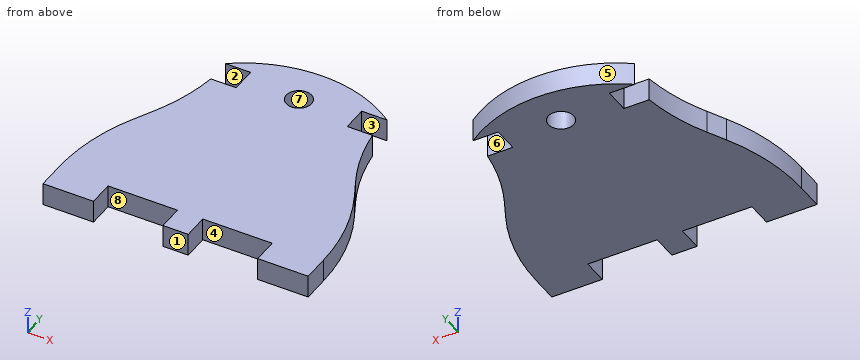
```python
from build123d import *

# Parameters (mm, degrees)
SKETCH1_R           = 2.5
BOSS_EXTRUDE1_DEPTH = 4.5
FILLET1_R           = 40
SKETCH2_W           = 5
SKETCH2_H           = 4.5
BOSS_EXTRUDE2_DEPTH = 5
CHAMFER1_SIZE       = 6
FILLET2_R           = 30
CUT_EXTRUDE1_DEPTH  = 10


# Some blends are built 0.0001 mm under size
with BuildPart() as part:
    # Sketch1 → Boss-Extrude1 (new body)
    with BuildSketch(Plane.XY):
        Polygon((-16.25, 10.704231142), (-16.25, 15.704231142), (16.25, 15.704231142), (16.25, 10.704231142), (26.25, 10.704231142), (26.25, 25.704231142), (16, 45.704231142), (16, 50.704231142), (11, 50.704231142), (11, 55.704231142), (16, 55.704231142), (16, 61.704231142), (-16, 61.704231142), (-16, 55.704231142), (-11, 55.704231142), (-11, 50.704231142), (-16, 50.704231142), (-16, 45.704231142), (-26.25, 25.704231142), (-26.25, 10.704231142), align=None)
        with Locations((0, 53.212370659)):
            Circle(SKETCH1_R, mode=Mode.SUBTRACT)
    extrude(amount=BOSS_EXTRUDE1_DEPTH)

    # Fillet1
    # the kernel refuses this fillet: 40 mm, written as the material it adds along each edge
    with BuildSketch(Plane(origin=(-16, 45.704231142, 0), x_dir=(0, 1, 0), z_dir=(0, 0, 1))) as fillet1_piece_1:
        with BuildLine():
            CenterArc((10.355860331, 39.639812816), FILLET1_R, 242.864860378, 19.440324463)
            Line((-7.887771306, 4.042482794), (0, 0))
            Line((0, 0), (5, 0))
        make_face()
    extrude(amount=4.5)
    with BuildSketch(Plane(origin=(16, 45.704231142, 0), x_dir=(0.4560907909103989, -0.8899332505568757, 0), z_dir=(0, 0, 1))) as fillet1_piece_2:
        with BuildLine():
            CenterArc((8.863329132, 40), FILLET1_R, 250.559675537, 19.440324463)
            Line((-4.449666253, 2.280453955), (0, 0))
            Line((0, 0), (8.863329132, 0))
        make_face()
    extrude(amount=4.5)
    # the kernel refuses this fillet: 40 mm, written as the material it takes off along each edge
    with BuildSketch(Plane(origin=(-26.25, 25.704231142, -24.132640175), x_dir=(0, -1, 0), z_dir=(0, 0, 1))) as fillet1_2_piece_1:
        with BuildLine():
            CenterArc((FILLET1_R * 0.241326401753, FILLET1_R), FILLET1_R, 242.864860378, 27.135139622)
            Line((-FILLET1_R * 0.214764389157, FILLET1_R * 0.110066749443), (0, 0))
            Line((0, 0), (FILLET1_R * 0.241326401753, 0))
        make_face()
    extrude(amount=52.765280351, mode=Mode.SUBTRACT)
    with BuildSketch(Plane(origin=(26.25, 25.704231142, -24.132640175), x_dir=(0, -1, 0), z_dir=(0, 0, 1))) as fillet1_2_piece_2:
        with BuildLine():
            CenterArc((FILLET1_R * 0.241326401753, -FILLET1_R), FILLET1_R, 90, 27.135139622)
            Line((-FILLET1_R * 0.214764389157, -FILLET1_R * 0.110066749443), (0, 0))
            Line((0, 0), (FILLET1_R * 0.241326401753, 0))
        make_face()
    extrude(amount=52.765280351, mode=Mode.SUBTRACT)

    # Sketch2 → Boss-Extrude2 (add)
    with BuildSketch(Plane.XZ.offset(-15.704231142)):
        with Locations((0, 2.25)):
            Rectangle(SKETCH2_W, SKETCH2_H)
    extrude(amount=BOSS_EXTRUDE2_DEPTH)

    # Chamfer1
    chamfer1_edges = [part.edges().sort_by_distance(p)[0] for p in [
        (16, 61.704231142, 2.25),
        (-16, 61.704231142, 2.25),
    ]]
    chamfer(chamfer1_edges, length=CHAMFER1_SIZE - 0.0001)  # a hair under: the kernel refuses the full size

    # Fillet2
    # the kernel refuses this fillet: 30 mm, written as the material it takes off along each edge
    with BuildSketch(Plane(origin=(10.0001, 61.704231142, -29.999916665), x_dir=(-1, 0, 0), z_dir=(0, 0, 1))) as fillet2_piece_1:
        with BuildLine():
            CenterArc((11.999966666, 30), FILLET2_R, 233.130420665, 36.869579335)
            Line((-5.9999, 5.9999), (-6.359897333, 5.519898))
            ThreePointArc((-6.359897333, 5.519898), (-3.424214069, 2.575685931), (-0.424264069, -0.424264069))
            Line((-0.424264069, -0.424264069), (0, -0.6))
            Line((0, -0.6), (11.999966666, -0.6))
            Line((11.999966666, -0.6), (11.999966666, 0))
        make_face()
    extrude(amount=64.499833329, mode=Mode.SUBTRACT)
    with BuildSketch(Plane(origin=(-10.0001, 61.704231142, -29.999916665), x_dir=(-0.7071067811865477, -0.7071067811865472, 0), z_dir=(0, 0, 1))) as fillet2_piece_2:
        with BuildLine():
            CenterArc((12.727945632, 29.698461239), FILLET2_R, 225, 36.869579335)
            Line((-8.485257803, 8.485257803), (-8.909521872, 8.060993735))
            Line((-8.909521872, 8.060993735), (-0.424264069, -0.424264069))
            Line((-0.424264069, -0.424264069), (0, -0.6))
            ThreePointArc((0, -0.6), (4.242569976, -0.6), (8.400283839, -0.593969225))
            Line((8.400283839, -0.593969225), (8.485139953, 0))
        make_face()
    extrude(amount=64.499833329, mode=Mode.SUBTRACT)

    # Sketch3 → Cut-Extrude1 (cut)
    with BuildSketch(Plane.XY.offset(4.5)):
        with BuildLine():
            ThreePointArc((-16, 55.704231142), (0, 60.96256169), (16, 55.704231142))
            ThreePointArc((16, 55.704231142), (0, 69.243827032), (-16, 55.704231142))
        make_face()
    extrude(amount=-CUT_EXTRUDE1_DEPTH, mode=Mode.SUBTRACT)


solid = part.part
```
Check sheet for the modelled part. Datum: model origin and axes. Units: mm. Face numbers are marked on the shaded views. A direction names the side the tool comes from. Coordinates: 2 decimals unless noted, no trailing zeros. Order: outer loops, then holes, each group sorted by start corner. A loop starts at its lowest first (then second) coordinate and runs counter-clockwise, first axis right, second up. Notation, with made-up numbers: (2.25, 47) -> (21.25, 47) arc R18 ccw to (21.25, 66) -> close; hole circle Ø1 at (66, 13.5). An arc over 180 degrees is marked (long way). Write item = value, one per line. Start each with the question number.
1) Go/stop test with flat-tipped pins: P1, Ø1.3, axis at x = -9, z = 2, coming from the -Y side; P2, Ø1.5, axis at y = 46.5, z = 2, coming from the +X side; P3, Ø2, axis at x = 14, z = 3.5, coming from the +Y side. Record where each tip stops, or that it passes through.
2) Access from +Z, -Z, +X, -X, +Y, -Y to the whole of each face (thin tool, end or side, straight path). Record for the marked faces 1, 2, 3 and 4.
3) Cross-section at B-B (z = 1.75). Enter the section's corners in (x, y), then the cut area to 3 significant figures.
4) Cross-section at D-D (x = -8). Enter the section's corners in (y, z), then the cut area to 3 significant figures.
5) Cross-section at A-A (x = 0). Enter the section's corners in (y, z).
6) Mould release check, pull along Y, two halves, no side actions. Record for the marked faces 5, 6, 7 and 8: +Y half, -Y half, draft (parallel to the pull), parting line (faces both ways), or undercut.
7) Cross-section at C-C (y = 35.5). Enter the section's corners in (x, z), then the cut area to 3 significant figures.
8) Material ranges on L1, parallel to Y at x = 0, z = 2.1; L2, parallel to Y at x = -12, z = 0.45; L3, parallel to X at y = 40.5, z = 2.95, recorded low to high.
Ans:
q1.P1 = 15.7
q1.P2 = 16.99
q1.P3 = 57.62
q2.face_1 = +Z, -Z, +X, -X, -Y
q2.face_2 = +Z, -Z, -X
q2.face_3 = +Z, -Z, +X
q2.face_4 = +Z, -Z, -Y
q3.outline = (-26.25, 10.7) -> (-16.25, 10.7) -> (-16.25, 15.7) -> (-2.5, 15.7) -> (-2.5, 10.7) -> (2.5, 10.7) -> (2.5, 15.7) -> (16.25, 15.7) -> (16.25, 10.7) -> (26.25, 10.7) -> (26.25, 16.05) arc R40 ccw to (21.85, 34.29) -> (20.04, 37.82) arc R40 cw to (16, 50.7) -> (11, 50.7) -> (11, 55.7) -> (16, 55.7) arc R26.97 ccw to (-16, 55.7) -> (-11, 55.7) -> (-11, 50.7) -> (-16, 50.7) arc R40 cw to (-20.04, 37.82) -> (-21.85, 34.29) arc R40 ccw to (-26.25, 16.05) -> close; hole circle Ø5 at (0, 53.21)
q3.area = 1,860 mm²
q4.outline = (15.7, 0) -> (59.75, 0) -> (59.75, 4.5) -> (15.7, 4.5) -> close
q4.area = 198 mm²
q5.outline = (10.7, 0) -> (50.71, 0) -> (50.71, 4.5) -> (10.7, 4.5) -> close; (55.71, 0) -> (60.96, 0) -> (60.96, 4.5) -> (55.71, 4.5) -> close
q6.face_5 = +Y half
q6.face_6 = undercut
q6.face_7 = undercut
q6.face_8 = -Y half
q7.outline = (-21.23, 0) -> (21.23, 0) -> (21.23, 4.5) -> (-21.23, 4.5) -> close
q7.area = 191 mm²
q8.L1 = 10.7 to 50.71, 55.71 to 60.96
q8.L2 = 15.7 to 50.7, 55.7 to 58.15
q8.L3 = -18.79 to 18.79
